Read the model definition and answer for the solid it produces. Units are mm, in the model's axes. A direction names the side the tool comes from. Coordinates: 2 decimals unless noted, no trailing zeros. Write each loop counter-clockwise with the first axis right and the second up, starting at its lowest first coordinate (ties: lowest second). Pieces come first, ordered by that corner, then holes. Notation, with made-up numbers: (29.5, 44.5) -> (63.5, 44.5) arc R17 cw to (63.5, 59.5) -> close; hole circle Ø3 at (57, -36). An arc over 180 degrees is marked (long way). Use CSV: the item, a comma, the result in double quotes.
from build123d import *

# Parameters (mm, degrees)
CROQUIS1_R              = 15
SALIENTE_EXTRUIR1_DEPTH = 50
SALIENTE_EXTRUIR2_START = 5
SALIENTE_EXTRUIR2_DEPTH = 5
CROQUIS3_R              = 1.5
CORTAR_EXTRUIR1_DEPTH   = 5
CORTAR_EXTRUIR2_DEPTH   = 25
SALIENTE_EXTRUIR3_START = 10
CROQUIS5_R              = 1.5
SALIENTE_EXTRUIR3_DEPTH = 5
CROQUIS6_R              = 22.280416197
CROQUIS6_R_2            = 15
CORTAR_EXTRUIR3_DEPTH   = 20


with BuildPart() as part:
    # Croquis1 → Saliente-Extruir1 (new body)
    with BuildSketch(Plane(origin=(0, 0, 0), x_dir=(1, 0, 0), z_dir=(0, 1, 0))):
        with Locations(Location((0, 0, 0), (0, 0, 270))):
            Circle(CROQUIS1_R)
    extrude(amount=SALIENTE_EXTRUIR1_DEPTH)

    # Croquis2 → Saliente-Extruir2 (add)
    with BuildSketch(Plane.XY.offset(SALIENTE_EXTRUIR2_START)):
        with BuildLine():
            Line((-8, 0), (-2.343145751, -5.656854249))
            ThreePointArc((-2.343145751, -5.656854249), (0, -6.627416998), (2.343145751, -5.656854249))
            Line((2.343145751, -5.656854249), (8, 0))
            Line((8, 0), (-8, 0))
        make_face()
    saliente_extruir2 = extrude(amount=SALIENTE_EXTRUIR2_DEPTH)

    # Croquis3 → Cortar-Extruir1 (cut)
    with BuildSketch(Plane.XY.offset(10)):
        with Locations((0, -3.313708499)):
            Circle(CROQUIS3_R)
    cortar_extruir1 = extrude(amount=-CORTAR_EXTRUIR1_DEPTH, mode=Mode.SUBTRACT)

    # Simetría1: Saliente-Extruir2, Cortar-Extruir1 across plane
    add(saliente_extruir2.mirror(Plane.XY))
    add(cortar_extruir1.mirror(Plane.XY), mode=Mode.SUBTRACT)

    # Croquis4 → Cortar-Extruir2 (cut, symmetric)
    with BuildSketch(Plane.XY):
        Polygon((-8, 0), (-15, 0), (-15, 10), align=None)
    cortar_extruir2 = extrude(amount=CORTAR_EXTRUIR2_DEPTH, both=True, mode=Mode.SUBTRACT)

    # Simetría2: Cortar-Extruir2 across plane
    add(cortar_extruir2.mirror(Plane.ZX.offset(25)), mode=Mode.SUBTRACT)

    # Croquis5 → Saliente-Extruir3 (add)
    with BuildSketch(Plane.XY.offset(SALIENTE_EXTRUIR3_START)):
        with BuildLine():
            Line((-8, 50), (-2.343145751, 55.656854249))
            ThreePointArc((-2.343145751, 55.656854249), (0, 56.627416998), (2.343145751, 55.656854249))
            Line((2.343145751, 55.656854249), (8, 50))
            Line((8, 50), (-8, 50))
        make_face()
        with Locations((0, 53.313708499)):
            Circle(CROQUIS5_R, mode=Mode.SUBTRACT)
    saliente_extruir3 = extrude(amount=SALIENTE_EXTRUIR3_DEPTH)

    # Simetría3: Saliente-Extruir3 across plane
    add(saliente_extruir3.mirror(Plane.XY))

    # Croquis6 → Cortar-Extruir3 (cut)
    with BuildSketch(Plane(origin=(0, 50, 0), x_dir=(1, 0, 0), z_dir=(0, 1, 0))):
        Circle(CROQUIS6_R)
        with Locations(Location((0, 0, 0), (0, 0, 122.230952636))):
            Circle(CROQUIS6_R_2, mode=Mode.SUBTRACT)
    extrude(amount=CORTAR_EXTRUIR3_DEPTH, mode=Mode.SUBTRACT)


solid = part.part
1. Each of these flat-tipped pins is pushed along its axis until it touches: pin 1 Ø3 at (x, y) = (-5.5, 15.5) entering from +Z; pin 2 Ø8 at (x, y) = (-11, 44.5) entering from +Z; pin 3 Ø4 at (x, y) = (-11, 40) entering from +Z; pin 4 Ø2.5 at (x, y) = (0, 53.31) entering from -Z. Where does it stop, or does it pass through?
Solutions:
pin 1,"stops at z = 14.46"
pin 2,"stops at z = 13.27"
pin 3,"stops at z = 12"
pin 4,"passes through"
2. A cutting plane is placed at B-B (z = 6.5). Give the vertices of the cut face in (x, y), and give its area (3 significant figures).
Solutions:
outline,"(-13.52, 7.88) -> (-8, 0) -> (-2.34, -5.66) arc R3.31 ccw to (2.34, -5.66) -> (8, 0) -> (13.52, 0) -> (13.52, 50) -> (-8, 50) -> (-13.52, 42.12) -> close; hole circle Ø3 at (0, -3.31)"
area,"1,360 mm^2"
3. A cutting plane is placed at C-C (z = 0). Give the vertices of the cut face in (x, y), and give its area (3 significant figures).
Solutions:
outline,"(-15, 10) -> (-8, 0) -> (15, 0) -> (15, 50) -> (-8, 50) -> (-15, 40) -> close"
area,"1,430 mm^2"
4. A tool of negligible diameter and unlimited length cuts with its end or side. For faces 1 (the flat face through (0, 51, 10)), 2 (the flat face through (0, -1, -5)), 3 (the flat face through (5, 53, -12)), from which of +Z, -Z, +X, -X, +Y, -Y can it reach the whole face along a straight path? Write none if from no direction.
Solutions:
face 1,"+X, -X, +Y"
face 2,"+X, -X, -Y"
face 3,"+Z, -Z, +X, +Y"
5. A cutting plane is placed at A-A (x = 0). Give the number of separate pieces and of enclosed holes in the cut face, and give its area (3 significant figures).
Solutions:
separate pieces,"5"
enclosed holes,"0"
area,"1,570 mm^2"
6. For a pull along Y with two mould halves and no side action, classify faces 4 (the cylindrical face through (-0.325, -4.778, 7.535)), 5 (the flat face through (-5, 53, 12)), 6 (the flat face through (-10.8, 4, 0.2)), 7 (the cylindrical face through (-0.325, -4.778, -7.535)) as pulls with the +Y half, pulls with the -Y half, needs draft (parallel to the pull), parting line crosses it, or undercut.
Solutions:
face 4,"undercut"
face 5,"pulls with the +Y half"
face 6,"pulls with the -Y half"
face 7,"undercut"
7. A cutting plane is placed at D-D (y = 20.5). Give the vertices of the cut face in (x, z).
Solutions:
outline,"circle Ø30 at (0, 0)"
8. Find the intervals of material crossed by line 1 along Y through (x, z) = (0, 6); line 2 along Y through (x, z) = (0, 11.95); line 3 along Z through (x, y) = (1, -1), in increasing order.
Solutions:
line 1,"y = -6.63 to -4.81, -1.81 to 50"
line 2,"y = 0 to 51.81, 54.81 to 56.63"
line 3,"z = -10 to -5, 5 to 10"
